```python
from build123d import *

# Parameters (mm, degrees)
SKETCH1_W                       = 76.2
SKETCH1_H                       = 44.45
SKETCH1_R                       = 14.2875
BOSS_EXTRUDE1_DEPTH             = 12.7
FILLET1_R                       = 3.175
SKETCH3_W                       = 69.85
SKETCH3_H                       = 19.05
CUT_EXTRUDE2_DEPTH              = 60.905780189
F_1_4_0_25_DIAMETER_HOLE1_D     = 6.35
F_1_4_0_25_DIAMETER_HOLE1_DEPTH = 5.08
F_1_4_0_25_DIAMETER_HOLE1_TIP   = 1.907732465


with BuildPart() as part:
    # Sketch1 → Boss-Extrude1 (new, symmetric)
    with BuildSketch(Plane.XY):
        Rectangle(SKETCH1_W, SKETCH1_H)
        with Locations((19.05, 3.175)):
            Circle(SKETCH1_R, mode=Mode.SUBTRACT)
    extrude(amount=BOSS_EXTRUDE1_DEPTH, both=True)

    # Fillet1
    fillet1_edges = [part.edges().sort_by_distance(p)[0] for p in [
        (38.1, -22.225, 0),
        (38.1, 22.225, 0),
    ]]
    fillet(fillet1_edges, radius=FILLET1_R)

    # Sketch3 → Cut-Extrude2 (cut, through all)
    with BuildSketch(Plane.XZ.offset(22.225)):
        Rectangle(SKETCH3_W, SKETCH3_H)
    extrude(amount=-CUT_EXTRUDE2_DEPTH, mode=Mode.SUBTRACT)

    # 1/4 (0.25) Diameter Hole1
    with Locations(Plane.ZY.offset(38.1)):
        with Locations((0, 6.35), (0, -12.7)):
            Hole(F_1_4_0_25_DIAMETER_HOLE1_D / 2, depth=F_1_4_0_25_DIAMETER_HOLE1_DEPTH)
            with Locations((0, 0, -(F_1_4_0_25_DIAMETER_HOLE1_DEPTH + F_1_4_0_25_DIAMETER_HOLE1_TIP / 2))):  # 118° drill point
                Cone(0, F_1_4_0_25_DIAMETER_HOLE1_D / 2, F_1_4_0_25_DIAMETER_HOLE1_TIP, mode=Mode.SUBTRACT)


solid = part.part
```
The model under review builds one solid part; all positions refer to its coordinate system, in mm. A direction names the side the tool comes from. Round coordinates to 2 decimals unless told otherwise and drop trailing zeros. Loops run counter-clockwise (first coordinate to the right, second up) from the corner with the lowest first, then second, coordinate; pieces in that order, holes last. Notation, with made-up numbers: (72, 66) -> (122, 66) arc R27 cw to (122, 101) -> close; hole circle Ø4 at (-40, 4). An arc over 180 degrees is marked (long way). Answer in a Markdown table with one row per item.
1) Consider section A-A, the plane x = 19.05. Write out the cut boundary in (y, z) (1 decimal).
Taken from the geometry:
| item | result |
|---|---|
| outline | (-22.2, -12.7) -> (-11.1, -12.7) -> (-11.1, -9.5) -> (-22.2, -9.5) -> close; (-22.2, 9.5) -> (-11.1, 9.5) -> (-11.1, 12.7) -> (-22.2, 12.7) -> close; (17.5, -12.7) -> (22.2, -12.7) -> (22.2, -9.5) -> (17.5, -9.5) -> close; (17.5, 9.5) -> (22.2, 9.5) -> (22.2, 12.7) -> (17.5, 12.7) -> close |
2) Draft analysis for pull direction X (two halves, no side actions). For faces 4 (the flat face through (-34.925, 0, 0)), 5 (the flat face through (-7, 22.225, -10)), 6 (the flat face through (38.1, 0, 0)), state which applies: pulls with the +X half, pulls with the -X half, needs draft (parallel to the pull), parting line crosses it, or undercut.
Taken from the geometry:
| item | result |
|---|---|
| face 4 | undercut |
| face 5 | needs draft |
| face 6 | pulls with the +X half |
3) Tool access review of faces 1 (the flat face through (34.925, 0, 0)), 2 (the cylindrical face through (37.195, 21.27, -0.178)), 3 (the cylindrical face through (-36.49, 9.027, -1.707)): name each direction out of +Z, -Z, +X, -X, +Y, -Y from which nothing blocks a thin tool from reaching the whole face with its end or side.
Taken from the geometry:
| item | result |
|---|---|
| face 1 | +Y, -Y |
| face 2 | +Z, -Z, +X, +Y |
| face 3 | -X |
4) Consider section C-C, the plane x = -23.5. Write out the cut boundary in (y, z) (3 decimals), plus the area to 3 significant figures.
Taken from the geometry:
| item | result |
|---|---|
| outline | (-22.225, -12.7) -> (22.225, -12.7) -> (22.225, -9.525) -> (-22.225, -9.525) -> close; (-22.225, 9.525) -> (22.225, 9.525) -> (22.225, 12.7) -> (-22.225, 12.7) -> close |
| area | 282 mm² |
5) Wall thickness on line 1 along Y through (x, z) = (-37.4, 0) (3 decimals); line 2 along Y through (x, z) = (19.05, -10.35) (1 decimal); line 3 along Z through (x, y) = (4, -17.5) (3 decimals): over which ranges is each line inside the solid? List them lowest first.
Taken from the geometry:
| item | result |
|---|---|
| line 1 | y = -22.225 to -15.875, -9.525 to 3.175, 9.525 to 22.225 |
| line 2 | y = -22.2 to -11.1, 17.5 to 22.2 |
| line 3 | z = -12.7 to -9.525, 9.525 to 12.7 |
6) For pin 1 Ø4 at (y, z) = (-12.7, 0) entering from -X (3 decimals), flat-tipped, find the tip position at first contact; note if it passes through.
Taken from the geometry:
| item | result |
|---|---|
| pin 1 | stops at x = 34.925 |
7) Consider section B-B, the plane z = 0. Write out the cut boundary in (x, y) (3 decimals), plus the area to 3 significant figures.
Taken from the geometry:
| item | result |
|---|---|
| outline | (-38.1, -22.225) -> (-34.925, -22.225) -> (-34.925, -15.875) -> (-38.1, -15.875) -> close; (-38.1, -9.525) -> (-34.925, -9.525) -> (-34.925, 3.175) -> (-38.1, 3.175) -> close; (-38.1, 9.525) -> (-34.925, 9.525) -> (-34.925, 22.225) -> (-38.1, 22.225) -> close; (34.925, -22.225) arc R3.175 ccw to (38.1, -19.05) -> (38.1, 19.05) arc R3.175 ccw to (34.925, 22.225) -> close |
| area | 238 mm² |
